Design review of the part shown in the three views and the two pictorial views. Dimensions are in mm from the part's minimum x, y and z. Round coordinates to 2 decimals unless told otherwise and drop trailing zeros. Order: outer loops, then holes, each group sorted by start corner. A loop starts at its lowest first (then second) coordinate and runs counter-clockwise, first axis right, second up. Notation, with made-up numbers: M 49.5,-26 L 77.5,-26 A22 ccw 77.5,-6 Z; hole C 58.5,-18 d8. An arc over 180 degrees is marked long. Write item = value, one per line. Start each with the question number.
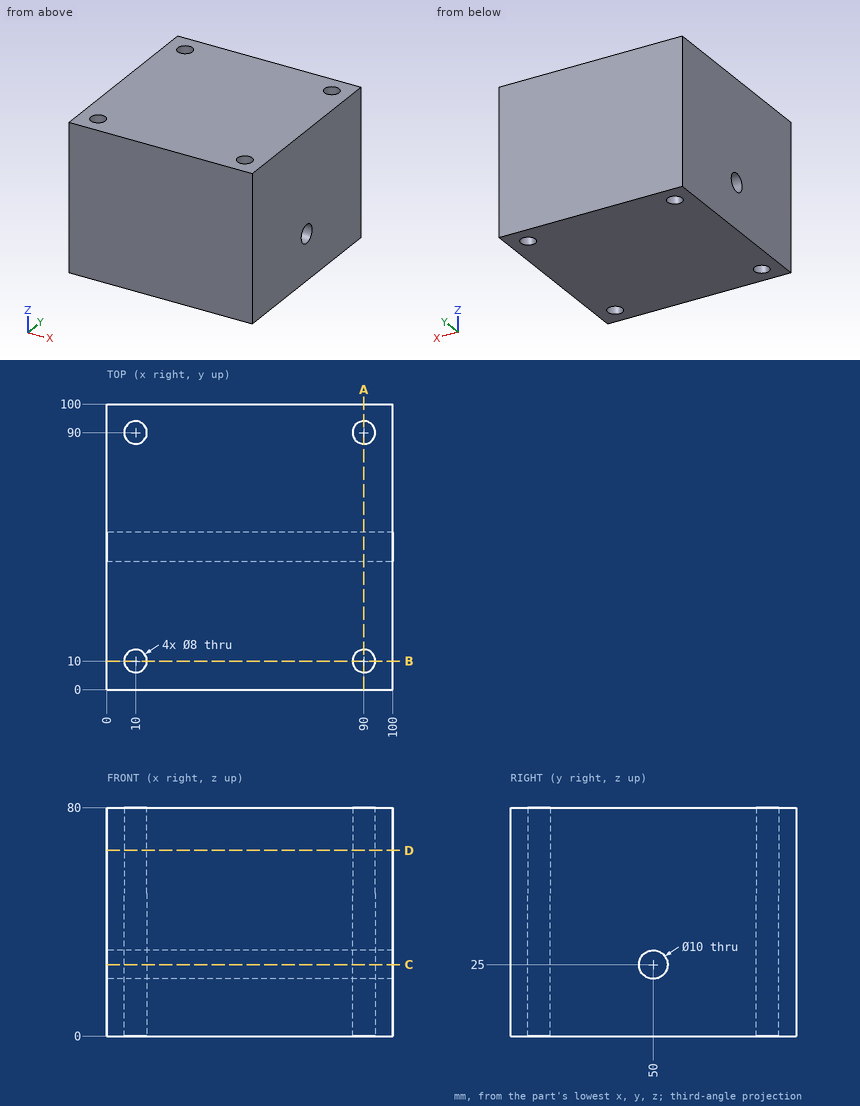
(1) We need section A-A, the plane x = 90. Write out the cut boundary in (y, z).
(2) We need section B-B, the plane y = 10. Write out the cut boundary in (x, z), then the cut area to 3 significant figures.
(3) For line 1 along Y through (x, z) = (10, 56); line 2 along X through (y, z) = (8.5, 54); line 3 along Z through (x, y) = (62, 50), list the stretches that pass through material, from the lowest coordinate up.
(4) We need section D-D, the plane z = 65. Write out the cut boundary in (x, y).
(5) Insertion check: pin 1 (5 mm diameter, centred on x = 90, y = 90, fed in from +Z). The pin has a flat end and moves straight along its axis. Give the tip position at first contact, or say it passes through.
(6) We need section C-C, the plane z = 25. Write out the cut boundary in (x, y).
Values:
q1.outline = M 0,0 L 6,0 L 6,80 L 0,80 Z; M 14,0 L 86,0 L 86,80 L 14,80 Z; M 94,0 L 100,0 L 100,80 L 94,80 Z; hole C 50,25 d10
q2.outline = M 0,0 L 6,0 L 6,80 L 0,80 Z; M 14,0 L 86,0 L 86,80 L 14,80 Z; M 94,0 L 100,0 L 100,80 L 94,80 Z
q2.area = 6,720 mm²
q3.line_1 = 0 to 6, 14 to 86, 94 to 100
q3.line_2 = 0 to 6.29, 13.71 to 86.29, 93.71 to 100
q3.line_3 = 0 to 20, 30 to 80
q4.outline = M 0,0 L 100,0 L 100,100 L 0,100 Z; hole C 10,10 d8; hole C 10,90 d8; hole C 90,10 d8; hole C 90,90 d8
q5.pin_1 = through
q6.outline = M 0,0 L 100,0 L 100,45 L 0,45 Z; M 0,55 L 100,55 L 100,100 L 0,100 Z; hole C 10,10 d8; hole C 10,90 d8; hole C 90,10 d8; hole C 90,90 d8
